Read the model definition and answer for the solid it produces. Units are mm, in the model's axes. Face numbers are marked on the shaded views. Coordinates: 2 decimals unless noted, no trailing zeros. Write each loop counter-clockwise with the first axis right and the second up, starting at its lowest first coordinate (ties: lowest second). Pieces come first, ordered by that corner, then holes. Notation, with made-up numbers: (35.25, 28) -> (59.25, 28) arc R14 ccw to (59.25, 40) -> close; hole circle Ø3 at (11.5, -8.75). An arc over 180 degrees is marked (long way). Use CSV: the item, a comma, the result in double quotes.
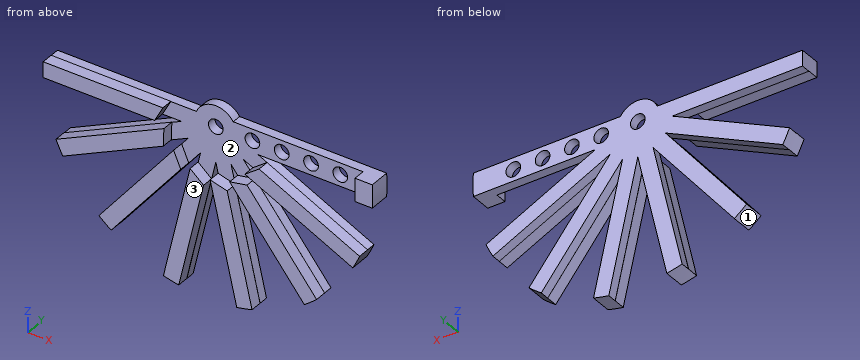
from build123d import *

# Parameters (mm, degrees)
SKETCH1_R           = 2
BOSS_EXTRUDE1_DEPTH = 2.54
BOSS_EXTRUDE2_DEPTH = 3.175
SKETCH4_W           = 8.755126744
SKETCH4_H           = 6.35
BOSS_EXTRUDE3_DEPTH = 3.175
SKETCH5_R           = 56.952437084
SKETCH5_R_2         = 45.011733307
CUT_EXTRUDE1_DEPTH  = 15.24


with BuildPart() as part:
    # Sketch1 → Boss-Extrude1 (new body)
    with BuildSketch(Plane(origin=(0, 0, 0), x_dir=(1, 0, 0), z_dir=(0, 1, 0))):
        with BuildLine():
            Line((-12.877451354, 48.231560826), (-17.055698858, 47.277903099))
            Line((-17.055698858, 47.277903099), (-8.251532809, 8.704331291))
            Line((-8.251532809, 8.704331291), (-32.920257894, 39.637934129))
            Line((-32.920257894, 39.637934129), (-36.270952237, 36.965844556))
            Line((-36.270952237, 36.965844556), (-11.602227151, 6.032241718))
            Line((-11.602227151, 6.032241718), (-47.249567728, 23.199096168))
            Line((-47.249567728, 23.199096168), (-49.109062801, 19.337814861))
            Line((-49.109062801, 19.337814861), (-13.461722225, 2.170960411))
            Line((-13.461722225, 2.170960411), (-53.027285305, 2.170960411))
            Line((-53.027285305, 2.170960411), (-53.027285305, -2.114738512))
            Line((-53.027285305, -2.114738512), (-9.372018351, -2.114738512))
            ThreePointArc((-9.372018351, -2.114738512), (-4.657137499, -5.657616121), (0.679371921, -3.14688905))
            Line((0.679371921, -3.14688905), (44.880714695, -3.14688905))
            Line((44.880714695, -3.14688905), (44.880714695, 0.02811095))
            Line((44.880714695, 0.02811095), (44.880714695, 3.20311095))
            Line((44.880714695, 3.20311095), (7.458434292, 3.20311095))
            Line((7.458434292, 3.20311095), (40.962492191, 19.337814861))
            Line((40.962492191, 19.337814861), (39.102997117, 23.199096168))
            Line((39.102997117, 23.199096168), (3.455656541, 6.032241718))
            Line((3.455656541, 6.032241718), (28.124381626, 36.965844556))
            Line((28.124381626, 36.965844556), (24.773687284, 39.637934129))
            Line((24.773687284, 39.637934129), (0.104962198, 8.704331291))
            Line((0.104962198, 8.704331291), (8.909128247, 47.277903099))
            Line((8.909128247, 47.277903099), (4.730880744, 48.231560826))
            Line((4.730880744, 48.231560826), (-4.073285305, 9.657989018))
            Line((-4.073285305, 9.657989018), (-12.877451354, 48.231560826))
        make_face()
        with Locations((-4.073285305, 0.02811095)):
            Circle(SKETCH1_R, mode=Mode.SUBTRACT)
        with Locations((5.926714695, 0.02811095)):
            Circle(SKETCH1_R, mode=Mode.SUBTRACT)
        with Locations((13.926714695, 0.02811095)):
            Circle(SKETCH1_R, mode=Mode.SUBTRACT)
        with Locations((21.926714695, 0.02811095)):
            Circle(SKETCH1_R, mode=Mode.SUBTRACT)
        with Locations((29.926714695, 0.02811095)):
            Circle(SKETCH1_R, mode=Mode.SUBTRACT)
    extrude(amount=BOSS_EXTRUDE1_DEPTH)

    # Sketch3 → Boss-Extrude2 (add)
    with BuildSketch(Plane.XZ):
        Polygon((40.962492191, -19.337814861), (39.102997117, -23.199096168), (6.04600763, -7.279689057), (9.932157206, -4.394393119), align=None)
        Polygon((6.638401546, -10.036078698), (28.111723935, -36.963461939), (24.76099628, -39.635509739), (1.885207385, -10.949444147), align=None)
        Polygon((1.222949052, -13.689887234), (8.885971689, -47.267642171), (4.707700409, -48.221195721), (-3.455809874, -12.450409084), align=None)
        Polygon((-5.241544906, -14.632097606), (-12.906660536, -48.209374817), (-17.08487237, -47.255560825), (-8.919132396, -11.485283116), align=None)
        Polygon((-11.474638084, -12.676083302), (-32.949638901, -39.602127989), (-36.300199991, -36.929871333), (-13.422623046, -8.245231717), align=None)
        Polygon((-16.241722503, -8.209278105), (-47.272988898, -23.150765598), (-49.132243282, -19.28936839), (-16.074261552, -3.372021857), align=None)
        Polygon((-18.598567057, -2.116435888), (-53.039640443, -2.113859702), (-53.039319873, 2.171839209), (-16.348829699, 2.169094767), align=None)
    extrude(amount=BOSS_EXTRUDE2_DEPTH)

    # Sketch4 → Boss-Extrude3 (add)
    with BuildSketch(Plane.XZ):
        with Locations((40.503151323, -0.02811095)):
            Rectangle(SKETCH4_W, SKETCH4_H)
    extrude(amount=BOSS_EXTRUDE3_DEPTH)

    # Sketch5 → Cut-Extrude1 (cut)
    with BuildSketch(Plane(origin=(0, 2.54, 0), x_dir=(1, 0, 0), z_dir=(0, 1, 0))):
        with Locations((-4.073285305, 0.02811095)):
            Circle(SKETCH5_R)
        with Locations((-4.073285305, 0.02811095)):
            Circle(SKETCH5_R_2, mode=Mode.SUBTRACT)
    extrude(amount=-CUT_EXTRUDE1_DEPTH, mode=Mode.SUBTRACT)


solid = part.part
1. For a pull along X with two mould halves and no side action, classify the marked faces 1, 2 and 3 as pulls with the +X half, pulls with the -X half, needs draft (parallel to the pull), parting line crosses it, or undercut.
Solutions:
face 1,"pulls with the -X half"
face 2,"undercut"
face 3,"needs draft"
2. A cutting plane is placed at D-D (x = 33.5). Give the vertices of the cut face in (y, z) (3 decimals), and give its area (3 significant figures).
Solutions:
outline,"(-3.175, -20.501) -> (2.54, -20.501) -> (2.54, -15.744) -> (-3.175, -15.744) -> close; (0, -3.203) -> (2.54, -3.203) -> (2.54, 3.147) -> (0, 3.147) -> close"
area,"43.3 mm^2"
3. Each of these flat-tipped pins is pushed along its axis until it touches: pin 1 Ø2 at (x, z) = (-27.5, -4) entering from +Y; pin 2 Ø4.5 at (x, z) = (5.93, -0.03) entering from -Y; pin 3 Ø1.6 at (x, y) = (-31, -2.5) entering from +Z; pin 4 Ø0.8 at (x, y) = (-36, 2) entering from -Z. Where does it stop, or does it pass through?
Solutions:
pin 1,"passes through"
pin 2,"stops at y = 0"
pin 3,"stops at z = 2.17"
pin 4,"stops at z = -17.97"
4. Find the intervals of material crossed by line 1 along X through (y, z) = (1.2, -0.5); line 2 along X through (y, z) = (-2.65, -24); line 3 along X through (y, z) = (-2.25, -29), in increasing order.
Solutions:
line 1,"x = -49.08 to -6.02, -2.13 to 3.98, 7.87 to 11.98, 15.87 to 19.98, 23.87 to 27.98, 31.87 to 40.94"
line 2,"x = -25.99 to -20.51, -11.78 to -7.38, -0.82 to 3.58, 12.29 to 17.77"
line 3,"x = -29.98 to -24.49, -12.92 to -8.52, 0.32 to 4.72, 16.28 to 21.76"
5. A cutting plane is placed at A-A (y = -1.75). Give the number of separate pieces and of enclosed holes in the cut face, and give its area (3 significant figures).
Solutions:
separate pieces,"8"
enclosed holes,"0"
area,"979 mm^2"
6. A cutting plane is placed at B-B (x = 17.5). Give the vertices of the cut face in (y, z) (3 decimals).
Solutions:
outline,"(-3.175, -30.53) -> (0, -30.53) -> (0, -30.517) -> (2.54, -30.517) -> (2.54, -23.643) -> (0, -23.643) -> (0, -23.656) -> (-3.175, -23.656) -> close; (-3.175, -12.796) -> (2.54, -12.796) -> (2.54, -8.039) -> (-3.175, -8.039) -> close; (0, -3.203) -> (2.54, -3.203) -> (2.54, 3.147) -> (0, 3.147) -> close"
